Here's how the part is built. I have some questions about the finished solid (model axes, mm). Give positions to 0.01 mm unless a question says otherwise; leave off trailing zeros. Loops run counter-clockwise (first coordinate to the right, second up) from the corner with the lowest first, then second, coordinate; pieces in that order, holes last. Notation, with made-up numbers: (32, 33) - (69, 33) arc R10 ccw to (69, 41) - close; hole circle Ø11 at (55.25, -9.75). An arc over 180 degrees is marked (long way). Return JSON: item names as keys, results as strings. Group by question number.
(1) I need wall thicknesses on probe 1 along Z at (x, y) = (8, 0.7); probe 2 along X at (y, z) = (4.75, -7.5); probe 3 along Z at (x, y) = (-22, 1.4). Which ranges of each line are inside material? Lowest first, please. Write a range as [from, to].
(2) If we section it at C-C (y = 3.15): Please give me the cut outline in (x, z).
(3) For P1, Ø1.5, axis at y = 4, z = -18.5, coming from the -X side; P2, Ø2, axis at x = 22.5, y = 4, coming from the +Z side; P3, Ø6.5, axis at x = -14.01, z = 0, coming from the +Y side, each with a flat end and sliding along its axis, tell me the tip position at first contact or that it passes through.
(4) If we section it at D-D (z = 52): Please give me the cut outline in (x, y), then the cut area to 3 significant figures.
(5) If we section it at A-A (z = 0): Please give me the cut outline in (x, y).
(6) If we section it at B-B (x = 0): Please give me the cut outline in (y, z).
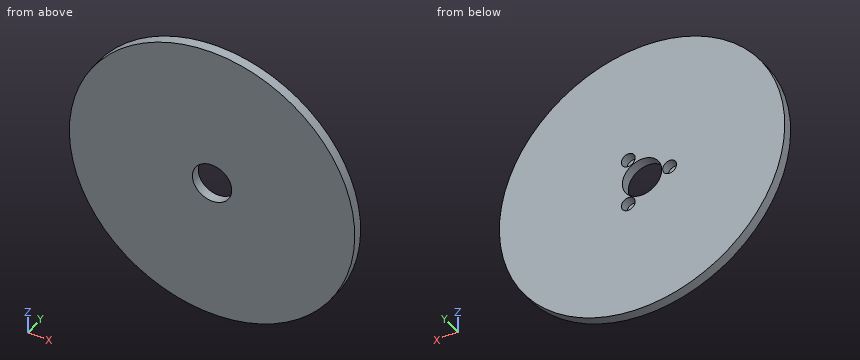
```python
from build123d import *

# Parameters (mm, degrees)
SKETCH1_R             = 72.5
BOSS_EXTRUDE1_DEPTH   = 5
SKETCH2_R             = 10
CUT_EXTRUDE1_DEPTH    = 103.652325838
SKETCH3_R             = 3.525017378
CUT_EXTRUDE2_DEPTH    = 4.708016
CIRPATTERN1_START     = 0.291983884
CIRPATTERN1_OUTLINE_R = 3.525017378
CIRPATTERN1_DEPTH     = 4.708016116


# Read off the part's stored shape, not the designer's step: CirPattern1
with BuildPart() as part:
    # Sketch1 → Boss-Extrude1 (new body)
    with BuildSketch(Plane(origin=(0, 0, 0), x_dir=(1, 0, 0), z_dir=(0, 1, 0))):
        with Locations(Location((0, 0, 0), (0, 0, 270))):
            Circle(SKETCH1_R)
    extrude(amount=BOSS_EXTRUDE1_DEPTH)

    # Sketch2 → Cut-Extrude1 (cut, through all)
    with BuildSketch(Plane(origin=(0, 0, 0), x_dir=(1, 0, 0), z_dir=(0, 1, 0))):
        with Locations(Location((0, 0, 0), (0, 0, 270))):
            Circle(SKETCH2_R)
    extrude(amount=CUT_EXTRUDE1_DEPTH, mode=Mode.SUBTRACT)

    # Sketch3 → Cut-Extrude2 (cut)
    with BuildSketch(Plane(origin=(0, 5, 0), x_dir=(1, 0, 0), z_dir=(0, 1, 0))):
        with Locations(Location((-14.005246001, 0, 0), (0, 0, 270))):
            Circle(SKETCH3_R)
    extrude(amount=-CUT_EXTRUDE2_DEPTH, mode=Mode.SUBTRACT)

    # CirPattern1 outline → CirPattern1 (cut)
    with BuildSketch(Plane(origin=(0, 0, 0), x_dir=(1, 0, 0), z_dir=(0, 1, 0)).offset(CIRPATTERN1_START)):
        with Locations((7.002623, 12.128898823)):
            Circle(CIRPATTERN1_OUTLINE_R)
        with Locations((7.002623, -12.128898823)):
            Circle(CIRPATTERN1_OUTLINE_R)
    extrude(amount=CIRPATTERN1_DEPTH, mode=Mode.SUBTRACT)


solid = part.part
```
Values:
{
 "1": {"probe 1": "[-72.06, -15.51], [-8.75, -6], [6, 8.75], [15.51, 72.06]", "probe 2": "[-72.11, -6.61], [6.61, 72.11]", "probe 3": "[-69.08, 69.08]"},
 "2": {"outline": "circle Ø145 at (0, 0); hole circle Ø7.05 at (-14.01, 0); hole circle Ø20 at (0, 0); hole circle Ø7.05 at (7, -12.13); hole circle Ø7.05 at (7, 12.13)"},
 "3": {"P1": "x = -70.29", "P2": "z = 69.24", "P3": "y = 0.29"},
 "4": {"outline": "(-50.52, 0) - (50.52, 0) - (50.52, 5) - (-50.52, 5) - close", "area": "505 mm2"},
 "5": {"outline": "(-72.5, 0) - (-10, 0) - (-10, 5) - (-10.48, 5) - (-10.48, 0.29) - (-17.53, 0.29) - (-17.53, 5) - (-72.5, 5) - close; (10, 0) - (72.5, 0) - (72.5, 5) - (10, 5) - close"},
 "6": {"outline": "(0, -72.5) - (5, -72.5) - (5, -10) - (0, -10) - close; (0, 10) - (5, 10) - (5, 72.5) - (0, 72.5) - close"}
}
